```python
from build123d import *

# Parameters (mm, degrees)
F0_W      = 711.2
F0_H      = 444.5
F0_W_2    = 660.4
F0_H_2    = 393.7
F1_DEPTH  = 215.9
F2_W      = 660.4
F2_H      = 165.1
F3_DEPTH  = 444.501
F4_W      = 393.7
F4_H      = 165.1
F5_DEPTH  = 711.201
F6_W      = 25.4
F6_H      = 25.4
F7_DEPTH  = 393.7
F8_W      = 25.4
F8_H      = 25.4
F9_DEPTH  = 393.7
F10_W     = 25.4
F10_H     = 25.4
F11_DEPTH = 165.1


with BuildPart() as f1:
    # F0 (on Top) → F1 (new body)
    with BuildSketch(Plane.XY):
        with Locations((355.6, 222.25)):
            Rectangle(F0_W, F0_H)
        with Locations((355.6, 222.25)):
            Rectangle(F0_W_2, F0_H_2, mode=Mode.SUBTRACT)
    extrude(amount=F1_DEPTH)

    # F2 (on face) → F3 (cut, through all)
    with BuildSketch(Plane.XZ):
        with Locations((355.6, 107.95)):
            Rectangle(F2_W, F2_H)
    extrude(amount=-F3_DEPTH, mode=Mode.SUBTRACT)

    # F4 (on face) → F5 (cut, through all)
    with BuildSketch(Plane.YZ.offset(711.2)):
        with Locations((222.25, 107.95)):
            Rectangle(F4_W, F4_H)
    extrude(amount=-F5_DEPTH, mode=Mode.SUBTRACT)

    # F6 (on face) → F7 (join, through all)
    with BuildSketch(Plane.XZ.offset(-419.1)):
        with Locations((215.9, 203.2)):
            Rectangle(F6_W, F6_H)
    extrude(amount=F7_DEPTH)

    # F8 (on face) → F9 (join, through all)
    with BuildSketch(Plane(origin=(0, 25.4, 0), x_dir=(-1, 0, 0), z_dir=(0, 1, 0))):
        with Locations((-215.9, 12.7)):
            Rectangle(F8_W, F8_H)
    extrude(amount=F9_DEPTH)

    # F10 (on face) → F11 (join, through all)
    with BuildSketch(Plane(origin=(0, 0, 190.5), x_dir=(1, 0, 0), z_dir=(0, 0, -1))):
        with Locations((215.9, -431.8)):
            Rectangle(F10_W, F10_H)
        with Locations((215.9, -12.7)):
            Rectangle(F10_W, F10_H)
    extrude(amount=F11_DEPTH)


solid = f1.part
```
CAD build for the part. Positions are in the model's coordinates, mm. A direction names the side the tool comes from. Round coordinates to 2 decimals unless told otherwise and drop trailing zeros. Write each loop counter-clockwise with the first axis right and the second up, starting at its lowest first coordinate (ties: lowest second). Pieces come first, ordered by that corner, then holes.
Item 1: Band-saw the part on C-C on x = 93.5. Write the cut outline in (y, z).
Filled in:
outline: (0, 0) - (25.4, 0) - (25.4, 25.4) - (0, 25.4) - close; (0, 190.5) - (25.4, 190.5) - (25.4, 215.9) - (0, 215.9) - close; (419.1, 0) - (444.5, 0) - (444.5, 25.4) - (419.1, 25.4) - close; (419.1, 190.5) - (444.5, 190.5) - (444.5, 215.9) - (419.1, 215.9) - close
Item 2: Band-saw the part on A-A on z = 98.5. Write the cut outline in (x, y), then the cut area to 3 significant figures.
Filled in:
outline: (0, 0) - (25.4, 0) - (25.4, 25.4) - (0, 25.4) - close; (0, 419.1) - (25.4, 419.1) - (25.4, 444.5) - (0, 444.5) - close; (203.2, 0) - (228.6, 0) - (228.6, 25.4) - (203.2, 25.4) - close; (203.2, 419.1) - (228.6, 419.1) - (228.6, 444.5) - (203.2, 444.5) - close; (685.8, 0) - (711.2, 0) - (711.2, 25.4) - (685.8, 25.4) - close; (685.8, 419.1) - (711.2, 419.1) - (711.2, 444.5) - (685.8, 444.5) - close
area: 3,870 mm2
Item 3: Drill centre lines: L1, parallel to X at y = 141.5, z = 204; L2, parallel to Z at x = 344, y = 423; L3, parallel to Y at x = 324.5, z = 196. Where is each one in solid material? Low to high.
Filled in:
L1: x = 0 to 25.4, 203.2 to 228.6, 685.8 to 711.2
L2: z = 0 to 25.4, 190.5 to 215.9
L3: y = 0 to 25.4, 419.1 to 444.5
Item 4: Tool access for faces 1 (the flat face through (454, 13, 190.5)), 2 (the flat face through (699, 25.4, 107)), 3 (the flat face through (685.8, 219, 13)): list every direction of +Z, -Z, +X, -X, +Y, -Y with a clear straight run to the whole face (end or side of a thin tool).
Filled in:
face 1: +Y, -Y
face 2: +X, -X
face 3: +Z, -Z
Item 5: Band-saw the part on B-B on y = 360.5. Write the cut outline in (x, z), then the cut area to 3 significant figures.
Filled in:
outline: (0, 0) - (25.4, 0) - (25.4, 25.4) - (0, 25.4) - close; (0, 190.5) - (25.4, 190.5) - (25.4, 215.9) - (0, 215.9) - close; (203.2, 0) - (228.6, 0) - (228.6, 25.4) - (203.2, 25.4) - close; (203.2, 190.5) - (228.6, 190.5) - (228.6, 215.9) - (203.2, 215.9) - close; (685.8, 0) - (711.2, 0) - (711.2, 25.4) - (685.8, 25.4) - close; (685.8, 190.5) - (711.2, 190.5) - (711.2, 215.9) - (685.8, 215.9) - close
area: 3,870 mm2
Item 6: Mould opens along Z. For faces 4 (the flat face through (222, 256, 0)), 5 (the flat face through (25.4, 432, 107)), 6 (the flat face through (228.6, 219, 13)) say: released by +Z, released by -Z, zero draft, split by the parting line, or undercut.
Filled in:
face 4: released by -Z
face 5: undercut
face 6: zero draft
